Work out the finished part from the listing and answer in its coordinate system (mm). A direction names the side the tool comes from. Round coordinates to 2 decimals unless told otherwise and drop trailing zeros. Loops run counter-clockwise (first coordinate to the right, second up) from the corner with the lowest first, then second, coordinate; pieces in that order, holes last. Notation, with made-up numbers: (-11.75, 11) - (27.25, 11) arc R10 ccw to (27.25, 16) - close; hole circle Ø8 at (31.25, 82.5). An arc over 180 degrees is marked (long way). Use CSV: the item, a comma, the result in double quotes. Start each with the question number.
from build123d import *

# Parameters (mm, degrees)
EXTRUDE_1_DEPTH      = 13
SKETCH_2_R           = 4
CUT_EXTRUDE_1_DEPTH  = 13
CUT_EXTRUDE_2_REACH  = 63.4
SKETCH_3_R           = 2.4
EXTRUDE_2_DEPTH      = 30
EXTRUDE_2_DEPTH_BACK = 13
SKETCH_4_R           = 4


with BuildPart() as part:
    # 草图1 → 凸台-拉伸1 (new body)
    with BuildSketch(Plane.XY):
        with BuildLine():
            Line((0, 0), (55, 0))
            Line((55, 0), (55, 5))
            Line((55, 5), (43.263269807, 5))
            Line((43.263269807, 5), (41.5, 15))
            ThreePointArc((41.5, 15), (27.5, 29), (13.5, 15))
            Line((13.5, 15), (11.736730193, 5))
            Line((11.736730193, 5), (0, 5))
            Line((0, 5), (0, 0))
        make_face()
    extrude(amount=EXTRUDE_1_DEPTH)

    # 草图2 → 切除-拉伸1 (cut)
    with BuildSketch(Plane.XY.offset(13)):
        with Locations((27.5, 15)):
            Circle(SKETCH_2_R)
    extrude(amount=-CUT_EXTRUDE_1_DEPTH, mode=Mode.SUBTRACT)

    # 草图3 → 切除-拉伸2 (cut, up to next)
    with BuildSketch(Plane(origin=(0, 5, 0), x_dir=(1, 0, 0), z_dir=(0, 1, 0)), mode=Mode.PRIVATE) as cut_extrude_2_sk1:
        with Locations(Location((6.5, -6.5, 0), (0, 0, 180))):
            Circle(SKETCH_3_R)
    cut_extrude_2_tool1 = extrude(cut_extrude_2_sk1.sketch, amount=-CUT_EXTRUDE_2_REACH, mode=Mode.PRIVATE) & part.part
    # 草图3 → 切除-拉伸2 (cut, up to next)
    with BuildSketch(Plane(origin=(0, 5, 0), x_dir=(1, 0, 0), z_dir=(0, 1, 0)), mode=Mode.PRIVATE) as cut_extrude_2_sk2:
        with Locations(Location((48.5, -6.5, 0), (0, 0, 180))):
            Circle(SKETCH_3_R)
    cut_extrude_2_tool2 = extrude(cut_extrude_2_sk2.sketch, amount=-CUT_EXTRUDE_2_REACH, mode=Mode.PRIVATE) & part.part
    add(cut_extrude_2_tool1.solids().sort_by_distance((6.5, 5, 6.5))[0], mode=Mode.SUBTRACT)
    add(cut_extrude_2_tool2.solids().sort_by_distance((48.5, 5, 6.5))[0], mode=Mode.SUBTRACT)

    # 草图4 → 凸台-拉伸2 (add, two sides: drawn at the far end of the back side and taken through both)
    with BuildSketch(Plane.XY.offset(13).offset(-EXTRUDE_2_DEPTH_BACK)):
        with Locations((27.5, 15)):
            Circle(SKETCH_4_R)
    extrude(amount=EXTRUDE_2_DEPTH + EXTRUDE_2_DEPTH_BACK)


solid = part.part
Item 1: The mould has two halves that part along Z. Classify faces 4 (the flat face through (3, 5, 6)), 5 (the cylindrical face through (50.898, 2.535, 6.606)), 6 (the flat face through (27, 15, 43)): pulls with the +Z half, pulls with the -Z half, needs draft (parallel to the pull), parting line crosses it, or undercut.
Item 2: Which of the six approach directions +Z, -Z, +X, -X, +Y, -Y give full straight-line access (tool end or side, diameter ignored) to faces 1 (the flat face through (51, 5, 5)), 2 (the cylindrical face through (24.55, 17.7, 27.79)), 3 (the flat face through (12.63, 10.07, 6.41))?
Item 3: A cutting plane is placed at B-B (x = 6.5). Determine the outline of the cut face in (y, z), plus the area to 3 significant figures.
Item 4: A cutting plane is placed at D-D (z = 21.5). Determine the outline of the cut face in (x, y).
Item 5: Find the intervals of material crossed by probe 1 along Z at (x, y) = (6.5, 2.55); probe 2 along Z at (x, y) = (39.5, 5.5); probe 3 along X at (y, z) = (16.5, 29.5), in increasing order. Write a range as [from, to].
Item 6: A cutting plane is placed at A-A (z = 8). Determine the outline of the cut face in (x, y), plus the area to 3 significant figures.
Item 7: Each of these flat-tipped pins is pushed along its axis until it touches: pin 1 Ø2 at (y, z) = (12, 33) entering from -X; pin 2 Ø6 at (x, z) = (47, 8.5) entering from +Y; pin 3 Ø2 at (y, z) = (8.5, 10) entering from -X. Where does it stop, or does it pass through?
Item 8: A cutting plane is placed at C-C (x = 27.5). Determine the outline of the cut face in (y, z).
Result sheet:
1,face 4,"needs draft"
1,face 5,"undercut"
1,face 6,"pulls with the +Z half"
2,face 1,"+Z, -Z, +X, +Y"
2,face 2,"+Z"
2,face 3,"+Z, -Z, -X, +Y"
3,outline,"(0, 0) - (5, 0) - (5, 4.1) - (0, 4.1) - close; (0, 8.9) - (5, 8.9) - (5, 13) - (0, 13) - close"
3,area,"41.0 mm^2"
4,outline,"circle Ø8 at (27.5, 15)"
5,probe 1,"[0, 4.1], [8.9, 13]"
5,probe 2,"[0, 13]"
5,probe 3,"[23.79, 31.21]"
6,outline,"(0, 0) - (4.63, 0) - (4.63, 5) - (0, 5) - close; (8.37, 0) - (46.63, 0) - (46.63, 5) - (43.26, 5) - (41.5, 15) arc R14 ccw to (13.5, 15) - (11.74, 5) - (8.37, 5) - close; (50.37, 0) - (55, 0) - (55, 5) - (50.37, 5) - close"
6,area,"843 mm^2"
7,pin 1,"x = 24.04"
7,pin 2,"y = 5"
7,pin 3,"x = 12.18"
8,outline,"(0, 0) - (29, 0) - (29, 13) - (19, 13) - (19, 43) - (11, 43) - (11, 13) - (0, 13) - close"
